from build123d import *

# Parameters (mm, degrees)
SKETCH_1_W          = 138.2
SKETCH_1_H          = 20
EXTRUDE_1_DEPTH     = 3
SKETCH_2_W          = 62
SKETCH_2_H          = 9.5
CUT_EXTRUDE_1_DEPTH = 3
SKETCH_3_W          = 16
SKETCH_3_H          = 20
EXTRUDE_2_DEPTH     = 1.5
FILLET_1_R          = 2


with BuildPart() as part:
    # 草图1 → 凸台-拉伸1 (new body)
    with BuildSketch(Plane(origin=(0, 0, 0), x_dir=(1, 0, 0), z_dir=(0, 1, 0))):
        with Locations((69.1, 10)):
            Rectangle(SKETCH_1_W, SKETCH_1_H)
    extrude(amount=EXTRUDE_1_DEPTH)

    # 草图2 → 切除-拉伸1 (cut)
    with BuildSketch(Plane(origin=(0, 3, 0), x_dir=(1, 0, 0), z_dir=(0, 1, 0))):
        with Locations((69.1, 15.25)):
            Rectangle(SKETCH_2_W, SKETCH_2_H)
    extrude(amount=-CUT_EXTRUDE_1_DEPTH, mode=Mode.SUBTRACT)

    # 草图3 → 凸台-拉伸2 (add)
    with BuildSketch(Plane(origin=(0, 3, 0), x_dir=(1, 0, 0), z_dir=(0, 1, 0))):
        with Locations((146.2, 10)):
            Rectangle(SKETCH_3_W, SKETCH_3_H)
        with Locations((-8, 10)):
            Rectangle(SKETCH_3_W, SKETCH_3_H)
    extrude(amount=-EXTRUDE_2_DEPTH)

    # 圆角1
    fillet_1_edges = [part.edges().sort_by_distance(p)[0] for p in [
        (154.2, 2.25, 0),
        (-16, 2.25, 0),
    ]]
    fillet(fillet_1_edges, radius=FILLET_1_R)


solid = part.part
Build history of the part. All positions in model axes, mm. A direction names the side the tool comes from. Round coordinates to 2 decimals unless told otherwise and drop trailing zeros. Write each loop counter-clockwise with the first axis right and the second up, starting at its lowest first coordinate (ties: lowest second). Pieces come first, ordered by that corner, then holes. Notation, with made-up numbers: (-6, 38.5) - (45, 38.5) arc R27 cw to (45, 68.5) - close; hole circle Ø11 at (-14.75, 43). An arc over 180 degrees is marked (long way). Use CSV: the item, a comma, the result in double quotes.
(1) Band-saw the part on D-D (x = 67.5). Write the cut outline in (y, z).
Response:
outline,"(0, -10.5) - (3, -10.5) - (3, 0) - (0, 0) - close"
(2) Pin check, flat tips, straight feed: P1, Ø1.2, axis at y = 0.5, z = -6, coming from the -X side; P2, Ø1.5, axis at x = 66.5, y = 1, coming from the -Z side; P3, Ø5, axis at x = -4.5, z = -6, coming from the -Y side. Stop position of each tip, or through.
Response:
P1,"x = 0"
P2,"z = -10.5"
P3,"y = 1.5"
(3) Wall check: line 1 (X direction, y = 1.3, z = -18.75); line 2 (X direction, y = 2.65, z = -17.75); line 3 (X direction, y = 0.25, z = -6.5). Give the ranges that are in metal, low to high.
Response:
line 1,"0 to 38.1, 100.1 to 138.2"
line 2,"-16 to 38.1, 100.1 to 154.2"
line 3,"0 to 138.2"
(4) Band-saw the part on C-C (z = -7.75). Write the cut outline in (x, y).
Response:
outline,"(-16, 1.5) - (0, 1.5) - (0, 0) - (138.2, 0) - (138.2, 1.5) - (154.2, 1.5) - (154.2, 3) - (-16, 3) - close"
(5) Band-saw the part on B-B (y = 2.55). Write the cut outline in (x, z), plus the area to 3 significant figures.
Response:
outline,"(-16, -20) - (38.1, -20) - (38.1, -10.5) - (100.1, -10.5) - (100.1, -20) - (154.2, -20) - (154.2, -2) arc R2 ccw to (152.2, 0) - (-14, 0) arc R2 ccw to (-16, -2) - close"
area,"2,810 mm²"
(6) 3-axis set-ups, long thin cutter, end or side, ignore diameter. For faces 1 (the flat face through (146, 1.5, -10)), 2 (the flat face through (38.1, 2, -15)), 3 (the flat face through (-8, 1.5, -10)): which of +Z, -Z, +X, -X, +Y, -Y reach the whole face in a straight line?
Response:
face 1,"+Z, -Z, +X, -Y"
face 2,"-Z, +Y, -Y"
face 3,"+Z, -Z, -X, -Y"
(7) Band-saw the part on A-A (z = -14). Write the cut outline in (x, y), plus the area to 3 significant figures.
Response:
outline,"(-16, 1.5) - (0, 1.5) - (0, 0) - (38.1, 0) - (38.1, 3) - (-16, 3) - close; (100.1, 0) - (138.2, 0) - (138.2, 1.5) - (154.2, 1.5) - (154.2, 3) - (100.1, 3) - close"
area,"277 mm²"
